Here's how the part is built. I have some questions about the finished solid (model axes, mm). Round coordinates to 2 decimals unless told otherwise and drop trailing zeros. Order: outer loops, then holes, each group sorted by start corner. A loop starts at its lowest first (then second) coordinate and runs counter-clockwise, first axis right, second up. Notation, with made-up numbers: (-27, 19.25) -> (-19, 19.25) arc R25 ccw to (-19, 31.25) -> close; hole circle Ø10 at (40, -25.5). An arc over 180 degrees is marked (long way). Use a Markdown table: item, result. Add a question column.
from build123d import *

# Parameters (mm, degrees)
F1_ANGLE_BACK = 120
F1_ANGLE      = 240
F3_DEPTH      = 200


with BuildPart() as f1:
    # F0 (on Right) → F1 (revolve)
    with BuildSketch(Plane.YZ, mode=Mode.PRIVATE) as f1_sk:
        with BuildLine():
            Line((0, 105), (0, 110))
            ThreePointArc((0, 110), (-55, 55), (0, 0))
            Line((0, 0), (0, 5))
            ThreePointArc((0, 5), (-50, 55), (0, 105))
        make_face()
    revolve(f1_sk.sketch.rotate(Axis((0, 0, 107.5), (0, 0, 1)), -F1_ANGLE_BACK), axis=Axis((0, 0, 107.5), (0, 0, 1)), revolution_arc=F1_ANGLE)

    # F2 (on face) → F3 (join)
    with BuildSketch(Plane(origin=(0, 0, 0), x_dir=(-0.8660254038, 0.5, 0), z_dir=(0.5, 0.8660254038, 0))):
        with BuildLine():
            ThreePointArc((0, 105), (50, 55), (0, 5))
            Line((0, 5), (0, 0))
            ThreePointArc((0, 0), (55, 55), (0, 110))
            Line((0, 110), (0, 105))
        make_face()
    extrude(amount=F3_DEPTH)


solid = f1.part
(1) I'm going to push flat-ended pins straight in: P1, Ø10, axis at x = 20, y = 133.5, coming from the -Z side; P2, Ø1.5, axis at x = 72, y = 130, coming from the -Z side; P3, Ø2, axis at y = 105, z = 35.5, coming from the +X side; P4, Ø10, axis at x = 61.5, y = -1, coming from the +Z side. Where does each tip first touch, or does it pass through?
(2) I want a section at A-A on z = 93.5. List the corners of the cut face in (x, y) for me.
(3) I want a section at B-B on x = 43.5. State how many separate pieces and enclosed holes the cut face has, and give its area (3 significant figures).
(4) I want a section at C-C on y = -28. List the corners of the cut face in (x, z) for me.
(5) Please list where these lines run through material, in increasing order: probe 1 along X at (y, z) = (-3.5, 91); probe 2 along Z at (x, y) = (35, 142); probe 3 along X at (y, z) = (13, 31). Write a range as from..to.
(6) I want a section at D-D on z = 28.5. List the corners of the cut face in (x, y) for me, and give its area (3 significant figures).
(7) If we mould it in two halves opening along Y, with no side actions, what happens to faces 1 (the cylindrical face through (1.68, 112.88, 53.79)), 2 (the cylindrical face through (6.009, 110.384, 56.099))? For each: pulls with the +Y half, pulls with the -Y half, needs draft (parallel to the pull), parting line crosses it, or undercut.
Output:
| question | item | result |
|---|---|---|
| 1 | P1 | z = 22.58 |
| 1 | P2 | z = 0.03 |
| 1 | P3 | x = 8.22 |
| 1 | P4 | through |
| 2 | outline | (-34.02, 19.64) arc R39.28 ccw (long way) to (34.02, 19.64) -> (27.63, 15.95) arc R31.9 cw (long way) to (-27.63, 15.95) -> (72.37, 189.16) -> (65.98, 192.84) -> close |
| 3 | separate pieces | 2 |
| 3 | enclosed holes | 1 |
| 3 | area | 3,040 mm² |
| 4 | outline | circle Ø94.68 at (0, 55); hole circle Ø82.85 at (0, 55) |
| 5 | probe 1 | -41.43..-34.52, 34.52..41.43 |
| 5 | probe 2 | 17.99..25.94, 84.06..92.01 |
| 5 | probe 3 | -47.75..-41.89, 41.89..47.75 |
| 6 | outline | (-41.74, 24.1) arc R48.19 ccw (long way) to (41.74, 24.1) -> (36.72, 21.2) arc R42.4 cw (long way) to (-36.72, 21.2) -> (63.28, 194.41) -> (58.26, 197.3) -> close |
| 6 | area | 2,260 mm² |
| 7 | face 1 | pulls with the +Y half |
| 7 | face 2 | undercut |
